Part print with two shaded views. Sizes in mm from the minimum x, y, z corner. A direction names the side the tool comes from. Coordinates: 2 decimals unless noted, no trailing zeros. Write each loop counter-clockwise with the first axis right and the second up, starting at its lowest first coordinate (ties: lowest second). Pieces come first, ordered by that corner, then holes.
Q1. Band-saw the part on A-A, the plane z = 10. Write the cut outline in (x, y), plus the area to 3 significant figures.
Q2. Band-saw the part on B-B, the plane x = 37.5. Write the cut outline in (y, z).
Q3. Band-saw the part on C-C, the plane y = 121.5. State how many separate pieces and enclosed holes the cut face has, plus the area to 3 significant figures.
Q4. Which spindle directions (+Z, -Z, +X, -X, +Y, -Y) get a long thin tool onto all of the face, cutting with end or side? Do the marked faces 1, 2 and 3. Say none if no direction does.
Q5. Pin check, flat tips, straight feed: P1, Ø10, axis at x = 40, y = 33.5, coming from the -Z side; P2, Ø10, axis at x = 13, z = 35, coming from the -Y side; P3, Ø2.5, axis at x = 23.5, z = 38.5, coming from the +Y side; P4, Ø10.5, axis at y = 123.5, z = 21, coming from the -X side. Stop position of each tip, or through.
Q6. Band-saw the part on D-D, the plane x = 43.5. Write the cut outline in (y, z), plus the area to 3 significant figures.
Q7. Pull direction X, two halves, no side cores. Call the marked faces 4, 5, 6 and 7: released by +X, released by -X, zero draft, split by the parting line, or undercut.
Q8. Drill centre lines: probe 1 along Z at (x, y) = (8.5, 2.75); probe 2 along X at (y, z) = (67.5, 16); probe 3 along Y at (x, z) = (13, 58). Where is each one in solid material? Low to high.
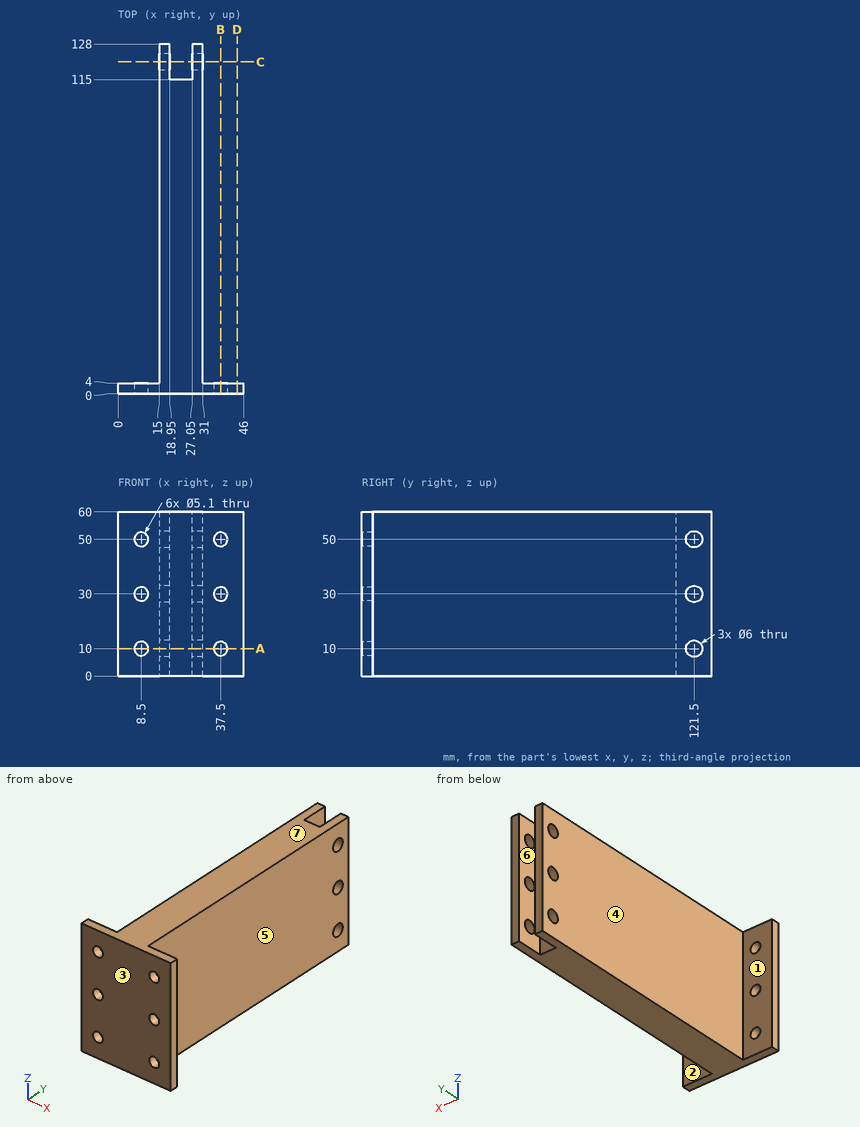
Answer sheet:
1. outline: (0, 0) - (5.95, 0) - (5.95, 4) - (0, 4) - close; (11.05, 0) - (34.95, 0) - (34.95, 4) - (31, 4) - (31, 118.5) - (27.05, 118.5) - (27.05, 115) - (18.95, 115) - (18.95, 118.5) - (15, 118.5) - (15, 4) - (11.05, 4) - close; (15, 124.5) - (18.95, 124.5) - (18.95, 128) - (15, 128) - close; (27.05, 124.5) - (31, 124.5) - (31, 128) - (27.05, 128) - close; (40.05, 0) - (46, 0) - (46, 4) - (40.05, 4) - close
1. area: 1,970 mm2
2. outline: (0, 0) - (4, 0) - (4, 7.45) - (0, 7.45) - close; (0, 12.55) - (4, 12.55) - (4, 27.45) - (0, 27.45) - close; (0, 32.55) - (4, 32.55) - (4, 47.45) - (0, 47.45) - close; (0, 52.55) - (4, 52.55) - (4, 60) - (0, 60) - close
3. separate pieces: 8
3. enclosed holes: 0
3. area: 332 mm2
4. face 1: +Z, -Z, -X, +Y
4. face 2: +Z, -Z, +X, +Y
4. face 3: +Z, -Z, +X, -X, -Y
5. P1: passes through
5. P2: stops at y = 0
5. P3: stops at y = 115
5. P4: stops at x = 15
6. outline: (0, 0) - (4, 0) - (4, 60) - (0, 60) - close
6. area: 240 mm2
7. face 4: released by -X
7. face 5: released by +X
7. face 6: undercut
7. face 7: zero draft
8. probe 1: z = 0 to 7.45, 12.55 to 27.45, 32.55 to 47.45, 52.55 to 60
8. probe 2: x = 15 to 31
8. probe 3: y = 0 to 4
